Source: three-view drawing plus pictorial views. Frame: mm from the lowest corner of the part. A direction names the side the tool comes from. Give positions to 0.01 mm unless a question says otherwise; leave off trailing zeros. Write each loop counter-clockwise with the first axis right and the second up, starting at its lowest first coordinate (ties: lowest second). Pieces come first, ordered by that corner, then holes.
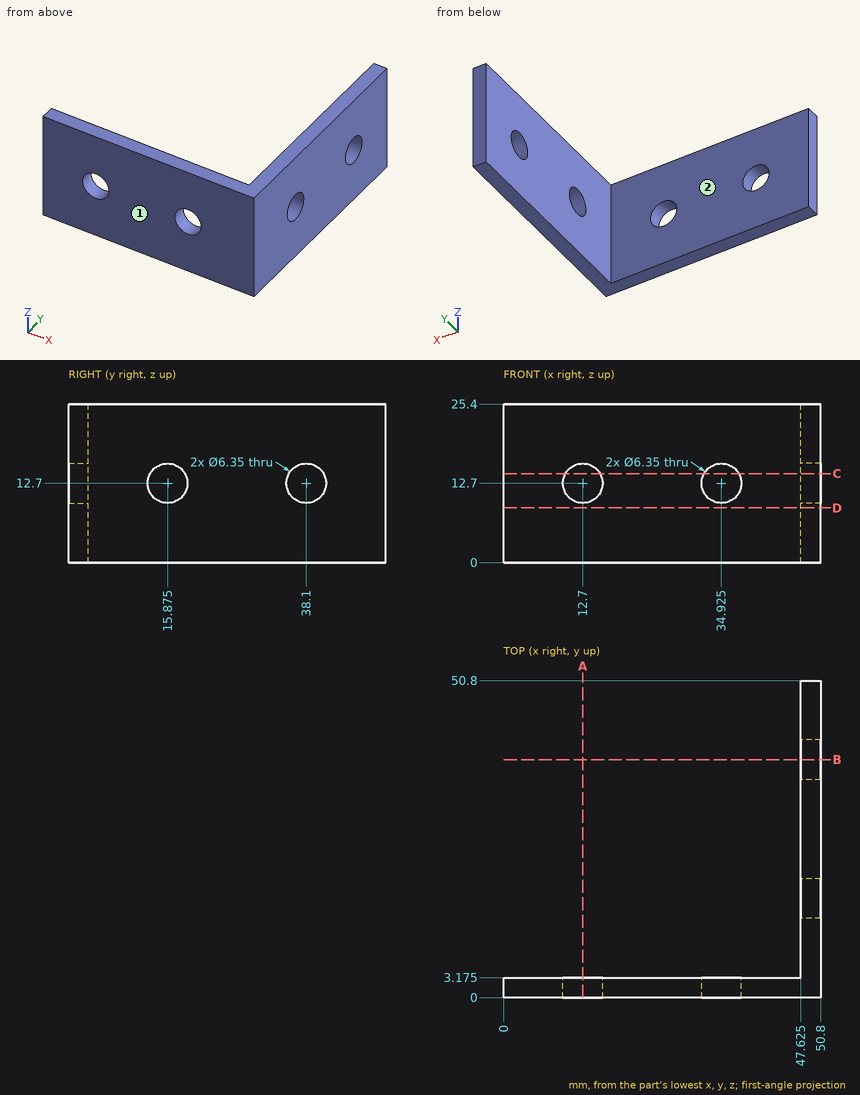
Q1. Access query for the marked faces 1 and 2. Directions: +Z, -Z, +X, -X, +Y, -Y. A direction counts if a zero-diameter tool reaches every point of the face in a straight line with its end or side. Return the directions, or none.
Filled sheet:
face 1: +Z, -Z, +X, -X, -Y
face 2: +Z, -Z, -X, +Y
Q2. Section D-D on z = 8.75. Output: boundary loops of the cut face in (x, y) (3 decimals), plus the area to 4 significant figures.
Filled sheet:
outline: (0, 0) - (50.8, 0) - (50.8, 50.8) - (47.625, 50.8) - (47.625, 3.175) - (0, 3.175) - close
area: 312.5 mm2
Q3. Ray query, line 1 along Y through (x, z) = (49.35, 12.7) (3 decimals); line 2 along X through (y, z) = (1.1, 12.7) (3 decimals); line 3 along Z through (x, y) = (48, 38). Return the intervals inside material, ascending.
Filled sheet:
line 1: y = 0 to 12.7, 19.05 to 34.925, 41.275 to 50.8
line 2: x = 0 to 9.525, 15.875 to 31.75, 38.1 to 50.8
line 3: z = 0 to 9.53, 15.87 to 25.4
Q4. Section B-B on y = 38.1. Output: boundary loops of the cut face in (x, z) (3 decimals), plus the area to 3 significant figures.
Filled sheet:
outline: (47.625, 0) - (50.8, 0) - (50.8, 9.525) - (47.625, 9.525) - close; (47.625, 15.875) - (50.8, 15.875) - (50.8, 25.4) - (47.625, 25.4) - close
area: 60.5 mm2
Q5. Section C-C on z = 14.25. Output: boundary loops of the cut face in (x, y) (3 decimals), plus the area to 3 significant figures.
Filled sheet:
outline: (0, 0) - (9.929, 0) - (9.929, 3.175) - (0, 3.175) - close; (15.471, 0) - (32.154, 0) - (32.154, 3.175) - (15.471, 3.175) - close; (37.696, 0) - (50.8, 0) - (50.8, 13.104) - (47.625, 13.104) - (47.625, 3.175) - (37.696, 3.175) - close; (47.625, 18.646) - (50.8, 18.646) - (50.8, 35.329) - (47.625, 35.329) - close; (47.625, 40.871) - (50.8, 40.871) - (50.8, 50.8) - (47.625, 50.8) - close
area: 242 mm2
Q6. Pin query (flat end, axial travel): P1, Ø6, axis at x = 13, z = 5, coming from the -Y side; P2, Ø4, axis at y = 12.5, z = 15.5, coming from the -X side (3 decimals). Return the tip coordinate at first contact, or that it passes through.
Filled sheet:
P1: stops at y = 0
P2: stops at x = 47.625
Q7. Section A-A on x = 12.7. Output: boundary loops of the cut face in (y, z) (3 decimals).
Filled sheet:
outline: (0, 0) - (3.175, 0) - (3.175, 9.525) - (0, 9.525) - close; (0, 15.875) - (3.175, 15.875) - (3.175, 25.4) - (0, 25.4) - close
